from build123d import *

# Parameters (mm, degrees)
F0_R        = 14.2875
F0_R_2      = 2.4892
F0_R_3      = 2.5527
F1_DEPTH    = 6.35
F2_R        = 12.7
F3_T1_DEPTH = 6.35


# Not quite as in the source:
# - a fillet or chamfer that OpenCascade refuses, or shapes differently, is made with other operations: its cross-section is extruded or revolved along the edge and cut away or added


with BuildPart() as f1:
    # F0 (on Front) → F1 (new body)
    with BuildSketch(Plane.XZ):
        with BuildLine():
            ThreePointArc((-73.767427816, -72.0958683029), (-74.7686667008, -74.2040007111), (-75.5037002278, -76.4190463696))
            ThreePointArc((-75.5037002278, -76.4190463696), (-76.040577327, -83.1861139792), (-74.1626528233, -89.7095211112))
            ThreePointArc((-74.1626528233, -89.7095211112), (-62.3780093009, -99.5325368374), (-47.1798914821, -97.4380976105))
            ThreePointArc((-47.1798914821, -97.4380976105), (-45.257025222, -96.0801463905), (-43.5169789975, -94.4946857926))
            ThreePointArc((-43.5169789975, -94.4946857926), (-39.5526914627, -88.4089490455), (-38.1635, -81.28))
            ThreePointArc((-38.1635, -81.28), (-39.1453760307, -75.2533344231), (-41.9894498038, -69.85))
            Line((-41.9894498038, -69.85), (-44.1945328452, -69.85))
            Line((-44.1945328452, -69.85), (-44.45, -69.85))
            Line((-44.45, -69.85), (-44.45, -67.1662768112))
            ThreePointArc((-44.45, -67.1662768112), (-45.5081692727, -66.2815014229), (-46.6277808452, -65.4758838808))
            ThreePointArc((-46.6277808452, -65.4758838808), (-54.8730151863, -62.430529917), (-63.6062431678, -63.4249137104))
            ThreePointArc((-63.6062431678, -63.4249137104), (-69.474566384, -66.8372770678), (-73.767427816, -72.0958683029))
        make_face()
        with Locations((-57.15, -81.28)):
            Circle(F0_R, mode=Mode.SUBTRACT)
        with BuildLine():
            Line((-44.45, -28.7643166542), (-44.45, -19.05))
            Line((-44.45, -19.05), (-73.767427816, -72.0958683029))
            ThreePointArc((-73.767427816, -72.0958683029), (-69.474566384, -66.8372770678), (-63.6062431678, -63.4249137104))
            Line((-63.6062431678, -63.4249137104), (-44.45, -28.7643166542))
        make_face()
        with BuildLine():
            Line((-75.5037002278, -76.4190463696), (-88.9, -127))
            Line((-88.9, -127), (-84.0389876487, -127))
            Line((-84.0389876487, -127), (-74.1626528233, -89.7095211112))
            ThreePointArc((-74.1626528233, -89.7095211112), (-76.040577327, -83.1861139792), (-75.5037002278, -76.4190463696))
        make_face()
        Polygon((-84.0389876487, -127), (-88.9, -127), (-88.9, -152.4), (0, -152.4), (0, -127), (-4.727917196, -127), (-17.3966372237, -127), (-23.4247913477, -127), (-61.7257976966, -127), (-68.1836898087, -127), align=None)
        with Locations((-76.2, -133.35)):
            Circle(F0_R_2, mode=Mode.SUBTRACT)
        with Locations((-63.5, -133.35)):
            Circle(F0_R_2, mode=Mode.SUBTRACT)
        with Locations((-50.8, -133.35)):
            Circle(F0_R_2, mode=Mode.SUBTRACT)
        with Locations((-38.1, -133.35)):
            Circle(F0_R_2, mode=Mode.SUBTRACT)
        with Locations((-25.4, -133.35)):
            Circle(F0_R_2, mode=Mode.SUBTRACT)
        with Locations((-12.7, -133.35)):
            Circle(F0_R_2, mode=Mode.SUBTRACT)
        Polygon((-4.727917196, -127), (0, -127), (-6.35, -69.85), (-11.077917196, -69.85), (-10.7374740973, -72.913987888), align=None)
        with BuildLine():
            Line((-6.35, -69.85), (-6.35, -19.05))
            Line((-6.35, -19.05), (-44.45, -19.05))
            Line((-44.45, -19.05), (-44.45, -28.7643166542))
            Line((-44.45, -28.7643166542), (-44.45, -62.9496581004))
            Line((-44.45, -62.9496581004), (-44.45, -67.1662768112))
            ThreePointArc((-44.45, -67.1662768112), (-43.7416474883, -67.8374085396), (-43.0687114356, -68.5440471649))
            ThreePointArc((-43.0687114356, -68.5440471649), (-42.5145067823, -69.1849795153), (-41.9894498038, -69.85))
            Line((-41.9894498038, -69.85), (-14.3068632521, -69.85))
            Line((-14.3068632521, -69.85), (-11.077917196, -69.85))
            Line((-11.077917196, -69.85), (-6.35, -69.85))
        make_face()
        with Locations((-38.1, -57.15)):
            Circle(F0_R_3, mode=Mode.SUBTRACT)
        with Locations((-25.4, -57.15)):
            Circle(F0_R_3, mode=Mode.SUBTRACT)
        with Locations((-12.7, -57.15)):
            Circle(F0_R_3, mode=Mode.SUBTRACT)
        with Locations((-38.1, -31.75)):
            Circle(F0_R_3, mode=Mode.SUBTRACT)
        with Locations((-25.4, -31.75)):
            Circle(F0_R_3, mode=Mode.SUBTRACT)
        with Locations((-12.7, -31.75)):
            Circle(F0_R_3, mode=Mode.SUBTRACT)
        Polygon((-44.0209157758, -101.3692673783), (-68.1836898087, -127), (-61.7257976966, -127), (-41.0492709397, -105.0673142856), align=None)
        Polygon((-40.7666595063, -97.9173056039), (-44.0209157758, -101.3692673783), (-41.0492709397, -105.0673142856), (-37.7950146701, -101.6153525111), align=None)
        Polygon((-10.7374740973, -72.913987888), (-11.077917196, -69.85), (-14.3068632521, -69.85), (-40.7666595063, -97.9173056039), (-37.7950146701, -101.6153525111), align=None)
        with BuildLine():
            Line((-47.1798914821, -97.4380976105), (-44.0209157758, -101.3692673783))
            Line((-44.0209157758, -101.3692673783), (-40.7666595063, -97.9173056039))
            Line((-40.7666595063, -97.9173056039), (-43.5169789975, -94.4946857926))
            ThreePointArc((-43.5169789975, -94.4946857926), (-45.257025222, -96.0801463905), (-47.1798914821, -97.4380976105))
        make_face()
        Polygon((-23.4247913477, -127), (-17.3966372237, -127), (-37.7950146701, -101.6153525111), (-41.0492709397, -105.0673142856), align=None)
        with BuildLine():
            ThreePointArc((-43.0687114356, -68.5440471649), (-43.7416474883, -67.8374085396), (-44.45, -67.1662768112))
            Line((-44.45, -67.1662768112), (-44.45, -69.85))
            Line((-44.45, -69.85), (-44.1945328452, -69.85))
            Line((-44.1945328452, -69.85), (-43.0687114356, -68.5440471649))
        make_face()
        with BuildLine():
            Line((-44.1945328452, -69.85), (-41.9894498038, -69.85))
            ThreePointArc((-41.9894498038, -69.85), (-42.5145067823, -69.1849795153), (-43.0687114356, -68.5440471649))
            Line((-43.0687114356, -68.5440471649), (-44.1945328452, -69.85))
        make_face()
    extrude(amount=F1_DEPTH)

    # F2
    f2_edges = [f1.edges().sort_by_distance(p)[0] for p in [
        (-6.35, -3.175, -19.05),
        (-88.9, -3.175, -152.4),
        (0, -3.175, -152.4),
        (-44.45, -3.175, -19.05),
    ]]
    fillet(f2_edges, radius=F2_R)

    # F3: fillet of radius 2.54 on 21 edges, made by hand

    # F3_s2 → F3_t1 (join)
    with BuildSketch(Plane.XZ):
        with BuildLine():
            ThreePointArc((-58.5225193342, -62.3431741591), (-60.8457611864, -61.1786129184), (-60.9292012272, -58.5811731507))
            Line((-60.9292012272, -58.5811731507), (-63.6062431678, -63.4249137104))
            ThreePointArc((-63.6062431678, -63.4249137104), (-61.1015719267, -62.7092633006), (-58.5225193342, -62.3431741591))
        make_face()
        with BuildLine():
            ThreePointArc((-42.2061934884, -92.9919524074), (-42.7469750096, -94.5742269942), (-42.1869747431, -96.1498021981))
            Line((-42.1869747431, -96.1498021981), (-43.5169789975, -94.4946857926))
            ThreePointArc((-43.5169789975, -94.4946857926), (-42.8418442978, -93.7605393574), (-42.2061934884, -92.9919524074))
        make_face()
        with BuildLine():
            ThreePointArc((-48.929563825, -98.3946607137), (-47.2679726242, -98.2071715059), (-45.8498872277, -99.0932140161))
            Line((-45.8498872277, -99.0932140161), (-47.1798914821, -97.4380976105))
            ThreePointArc((-47.1798914821, -97.4380976105), (-48.0421609425, -97.9393652326), (-48.929563825, -98.3946607137))
        make_face()
        with BuildLine():
            ThreePointArc((-71.2393441045, -94.007040699), (-73.7227097824, -93.2411748511), (-75.5795507042, -95.0593600393))
            Line((-75.5795507042, -95.0593600393), (-74.1626528233, -89.7095211112))
            ThreePointArc((-74.1626528233, -89.7095211112), (-72.8487490545, -91.958785529), (-71.2393441045, -94.007040699))
        make_face()
        with BuildLine():
            ThreePointArc((-44.45, -38.6110805765), (-46.35556752, -36.1515896884), (-49.2130672664, -37.3824341956))
            Line((-49.2130672664, -37.3824341956), (-44.45, -28.7643166542))
            Line((-44.45, -28.7643166542), (-44.45, -38.6110805765))
        make_face()
        with BuildLine():
            ThreePointArc((-38.7656990781, -95.7947810274), (-40.7142143439, -96.5904542384), (-42.5938492637, -95.6434694613))
            Line((-42.5938492637, -95.6434694613), (-40.7666595063, -97.9173056039))
            Line((-40.7666595063, -97.9173056039), (-38.7656990781, -95.7947810274))
        make_face()
        with BuildLine():
            ThreePointArc((-67.4317191857, -126.2023449812), (-68.2734267993, -126.7920759263), (-69.2799166769, -127))
            Line((-69.2799166769, -127), (-68.1836898087, -127))
            Line((-68.1836898087, -127), (-67.4317191857, -126.2023449812))
        make_face()
        with BuildLine():
            ThreePointArc((-80.7386977088, -127), (-82.7515748526, -126.0091693271), (-83.1940422209, -123.8097051999))
            Line((-83.1940422209, -123.8097051999), (-84.0389876487, -127))
            Line((-84.0389876487, -127), (-80.7386977088, -127))
        make_face()
        with BuildLine():
            ThreePointArc((-20.1921413698, -69.85), (-17.8600654435, -71.3835101223), (-18.3439438786, -74.1323449812))
            Line((-18.3439438786, -74.1323449812), (-14.3068632521, -69.85))
            Line((-14.3068632521, -69.85), (-20.1921413698, -69.85))
        make_face()
        with BuildLine():
            ThreePointArc((-45.4063150305, -99.6452149726), (-44.8482495326, -101.3365661623), (-45.5380702337, -102.9785933689))
            Line((-45.5380702337, -102.9785933689), (-44.0209157758, -101.3692673783))
            Line((-44.0209157758, -101.3692673783), (-45.4063150305, -99.6452149726))
        make_face()
        with BuildLine():
            ThreePointArc((-43.0502313678, -107.1898388621), (-41.1017161021, -106.394165651), (-39.2220811823, -107.3411504281))
            Line((-39.2220811823, -107.3411504281), (-41.0492709397, -105.0673142856))
            Line((-41.0492709397, -105.0673142856), (-43.0502313678, -107.1898388621))
        make_face()
        with BuildLine():
            ThreePointArc((-36.2778602123, -100.0060265206), (-36.9676809133, -101.6480537272), (-36.4096154155, -103.3394049169))
            Line((-36.4096154155, -103.3394049169), (-37.7950146701, -101.6153525111))
            Line((-37.7950146701, -101.6153525111), (-36.2778602123, -100.0060265206))
        make_face()
        with BuildLine():
            ThreePointArc((-57.68871707, -122.7176550188), (-58.1725955051, -125.4664898777), (-55.8405195788, -127))
            Line((-55.8405195788, -127), (-61.7257976966, -127))
            Line((-61.7257976966, -127), (-57.68871707, -122.7176550188))
        make_face()
        with BuildLine():
            ThreePointArc((-26.7443717706, -122.8689665849), (-26.4338196217, -125.5578103492), (-28.724324465, -127))
            Line((-28.724324465, -127), (-23.4247913477, -127))
            Line((-23.4247913477, -127), (-26.7443717706, -122.8689665849))
        make_face()
        with BuildLine():
            ThreePointArc((-5.0413056489, -124.1795039238), (-5.6731451696, -126.1539805144), (-7.565770335, -127))
            Line((-7.565770335, -127), (-4.727917196, -127))
            Line((-4.727917196, -127), (-5.0413056489, -124.1795039238))
        make_face()
        with BuildLine():
            ThreePointArc((-14.5038036224, -76.9091328532), (-11.8502584516, -76.2425330207), (-10.1311414451, -78.3709817581))
            Line((-10.1311414451, -78.3709817581), (-10.7374740973, -72.913987888))
            Line((-10.7374740973, -72.913987888), (-14.5038036224, -76.9091328532))
        make_face()
        with BuildLine():
            ThreePointArc((-16.1792469636, -127), (-17.2770573128, -126.7505048433), (-18.159199658, -126.0510334151))
            Line((-18.159199658, -126.0510334151), (-17.3966372237, -127))
            Line((-17.3966372237, -127), (-16.1792469636, -127))
        make_face()
        with BuildLine():
            ThreePointArc((-39.8582276098, -73.4389675516), (-39.6798917034, -71.0139145341), (-37.5449470225, -69.85))
            Line((-37.5449470225, -69.85), (-41.9894498038, -69.85))
            ThreePointArc((-41.9894498038, -69.85), (-40.8249124862, -71.5857388153), (-39.8582276098, -73.4389675516))
        make_face()
        with BuildLine():
            ThreePointArc((-44.45, -62.3019968846), (-45.6848952053, -64.4810566531), (-48.188820059, -64.5412892876))
            ThreePointArc((-48.188820059, -64.5412892876), (-46.2401732835, -65.7409246328), (-44.45, -67.1662768112))
            Line((-44.45, -67.1662768112), (-44.45, -62.3019968846))
        make_face()
    extrude(amount=F3_T1_DEPTH)


solid = f1.part
CAD build for the part. Positions are in the model's coordinates, mm. A direction names the side the tool comes from. Coordinates: 2 decimals unless noted, no trailing zeros. Write each loop counter-clockwise with the first axis right and the second up, starting at its lowest first coordinate (ties: lowest second). Pieces come first, ordered by that corner, then holes. Notation, with made-up numbers: M -31,-6 L 8,-6 A22 cw 8,25 Z; hole C 48.5,19.5 d1. An arc over 180 degrees is marked long. Return JSON: item names as keys, results as strings.
Item 1: Slice it at C-C, the plane z = -116. Write the cut outline in (x, y), and give its area (3 significant figures).
Findings below:
{"outline": "M -85.99,-6.35 L -81.13,-6.35 L -81.13,0 L -85.99,0 Z; M -57.81,-6.35 L -51.36,-6.35 L -51.36,0 L -57.81,0 Z; M -32.26,-6.35 L -26.24,-6.35 L -26.24,0 L -32.26,0 Z; M -5.95,-6.35 L -1.22,-6.35 L -1.22,0 L -5.95,0 Z", "area": "140 mm2"}
Item 2: Probe line 1 (X direction, y = -4, z = -55); line 2 (Z direction, x = -38.1, y = -3.5); line 3 (X direction, y = -5, z = -126). List the from-to ranges inside material, lowest first. Write a range as from..to.
Findings below:
{"line 1": "x = -64.32..-58.95, -44.45..-39.48, -36.72..-26.78, -24.02..-14.08, -11.32..-6.35", "line 2": "z = -152.4..-135.84, -130.86..-127, -108.74..-95.09, -69.91..-59.7, -54.6..-34.3, -29.2..-19.1", "line 3": "x = -88.64..-82.76, -67.24..-57.86, -26.7..-18.2, -5.55..-0.11"}
Item 3: Slice it at B-B, the plane x = -50.8. Write the cut outline in (y, z).
Findings below:
{"outline": "M -6.35,-152.4 L 0,-152.4 L 0,-135.84 L -6.35,-135.84 Z; M -6.35,-130.86 L 0,-130.86 L 0,-127 L -6.35,-127 Z; M -6.35,-115.41 L 0,-115.41 L 0,-108.56 L -6.35,-108.56 Z; M -6.35,-99.17 L 0,-99.17 L 0,-94.08 L -6.35,-94.08 Z; M -6.35,-68.48 L 0,-68.48 L 0,-63.39 L -6.35,-63.39 Z; M -6.35,-40.25 L 0,-40.25 L 0,-30.54 L -6.35,-30.54 Z"}
Item 4: Slice it at D-D, the plane x = -63.5. Write the cut outline in (y, z).
Findings below:
{"outline": "M -6.35,-152.4 L 0,-152.4 L 0,-135.84 L -6.35,-135.84 Z; M -6.35,-130.86 L 0,-130.86 L 0,-122.03 L -6.35,-122.03 Z; M -6.35,-99.17 L 0,-99.17 L 0,-94.08 L -6.35,-94.08 Z; M -6.35,-68.48 L 0,-68.48 L 0,-53.52 L -6.35,-53.52 Z"}
Item 5: Slice it at A-A, the plane z = -42.5. Write the cut outline in (x, y), and give its area (3 significant figures).
Findings below:
{"outline": "M -57.41,-6.35 L -52.04,-6.35 L -52.04,0 L -57.41,0 Z; M -44.45,-6.35 L -6.35,-6.35 L -6.35,0 L -44.45,0 Z", "area": "276 mm2"}
Item 6: Which spindle directions (+Z, -Z, +X, -X, +Y, -Y) get a long thin tool onto all of the face, cutting with end or side? Do faces 1 (the flat face through (-55.153, -3.131, -48.13)), 2 (the flat face through (-3.13, -3.13, -98.83)). Say none if no direction does.
Findings below:
{"face 1": "+Y, -Y", "face 2": "+Z, +X, +Y, -Y"}
Item 7: Drop flat-ended pins along their axis: pin 1 Ø1.9 at (x, y) = (-14, -4.5) entering from +Z; pin 2 Ø1.5 at (x, y) = (-45.5, -3) entering from +Z; pin 3 Ø3 at (x, y) = (-74, -4.5) entering from +Z. Give the stop position or say it passes through.
Findings below:
{"pin 1": "stops at z = -19.73", "pin 2": "stops at z = -21.72", "pin 3": "stops at z = -69.8"}
Item 8: Two-plate mould, pull along X, no slides. Class faces 3 (the flat face through (-88.9, -3, -133)), 4 (the cylindrical face through (-53.126, -3.131, -62.725)), 5 (the cylindrical face through (-9.97, -3.22, -22.87)): +X half, -X half, draft (parallel to the pull), parting line (faces both ways), or undercut.
Findings below:
{"face 3": "-X half", "face 4": "undercut", "face 5": "+X half"}
